Read the model definition and answer for the solid it produces. Units are mm, in the model's axes. A direction names the side the tool comes from. Coordinates: 2 decimals unless noted, no trailing zeros. Order: outer loops, then holes, each group sorted by start corner. A loop starts at its lowest first (then second) coordinate and runs counter-clockwise, first axis right, second up. Notation, with made-up numbers: (23, 85) - (50, 85) arc R17 ccw to (50, 108) - close; hole circle Ø1 at (-22.5, 69). An arc over 180 degrees is marked (long way). Write item = value, one per line.
from build123d import *

# Parameters (mm, degrees)
SKETCH1_W           = 25.9
SKETCH1_H           = 30
BOSS_EXTRUDE1_DEPTH = 7
BOSS_EXTRUDE2_DEPTH = 10
CUT_EXTRUDE1_DEPTH  = 10
SKETCH4_W           = 25.9
SKETCH4_H           = 7
BOSS_EXTRUDE3_DEPTH = 12


with BuildPart() as part:
    # Sketch1 → Boss-Extrude1 (new body)
    with BuildSketch(Plane.XY):
        with Locations((-0.908401305, 7.099021207)):
            Rectangle(SKETCH1_W, SKETCH1_H)
    extrude(amount=BOSS_EXTRUDE1_DEPTH)

    # Sketch2 → Boss-Extrude2 (add)
    with BuildSketch(Plane(origin=(0, 22.099021207, 0), x_dir=(1, 0, 0), z_dir=(0, 1, 0))):
        Polygon((-13.858401305, -4.5), (-16.158401305, -5.116283143), (-16.158401305, -1.733716857), (-13.858401305, -2.35), align=None)
        Polygon((12.041598695, -2.35), (14.341598695, -1.733716857), (14.341598695, -5.116283143), (12.041598695, -4.5), align=None)
    extrude(amount=-BOSS_EXTRUDE2_DEPTH)

    # Sketch3 → Cut-Extrude1 (cut)
    with BuildSketch(Plane(origin=(0, 0, 0), x_dir=(-1, 0, 0), z_dir=(0, 0, -1))):
        with BuildLine():
            Line((-3.791598695, 10.666053203), (-3.791598695, 22.099021207))
            Line((-3.791598695, 22.099021207), (5.608401305, 22.099021207))
            Line((5.608401305, 22.099021207), (5.608401305, 10.666053203))
            ThreePointArc((5.608401305, 10.666053203), (0.908401305, 5.966053203), (-3.791598695, 10.666053203))
        make_face()
    extrude(amount=-CUT_EXTRUDE1_DEPTH, mode=Mode.SUBTRACT)

    # Sketch4 → Boss-Extrude3 (add)
    with BuildSketch(Plane.XZ.offset(7.900978793)):
        with Locations((-0.908401305, 3.5)):
            Rectangle(SKETCH4_W, SKETCH4_H)
    extrude(amount=BOSS_EXTRUDE3_DEPTH)


solid = part.part
1) The part is cut by section C-C (z = 0.5). Determine the outline of the cut face in (x, y), and give its area (3 significant figures).
Returned:
outline = (-13.86, -19.9) - (12.04, -19.9) - (12.04, 22.1) - (3.79, 22.1) - (3.79, 10.67) arc R4.7 cw to (-5.61, 10.67) - (-5.61, 22.1) - (-13.86, 22.1) - close
area = 946 mm^2
2) For faces 5 (the face through (-5.608, 16, 3)), 6 (the face through (-15, 12.099, 3)), 7 (the face through (13.175, 17.169, 2.046)), 8 (the face through (-1, 1, 0)), 9 (the face through (13.208, 17.169, 4.812)), determine the directions among +Z, -Z, +X, -X, +Y, -Y from which every point of the face is accessible in a straight line to the end or side of a thin tool.
Returned:
face_5 = +Z, -Z, +Y
face_6 = +Z, -Z, -X, -Y
face_7 = -Z, +Y, -Y
face_8 = -Z, +X, -X, +Y, -Y
face_9 = +Z, +Y, -Y
3) Determine the mould class of faces 1 (the face through (14.342, 17, 3)), 2 (the face through (-16.158, 17, 3)), 3 (the face through (13, 12.099, 3)), 4 (the face through (3.792, 16, 3)) for opening direction X: pulls with the +X half, pulls with the -X half, needs draft (parallel to the pull), parting line crosses it, or undercut.
Returned:
face_1 = pulls with the +X half
face_2 = pulls with the -X half
face_3 = needs draft
face_4 = undercut
4) The part is cut by section B-B (y = -10). Determine the outline of the cut face in (x, z), and give its area (3 significant figures).
Returned:
outline = (-13.86, 0) - (12.04, 0) - (12.04, 7) - (-13.86, 7) - close
area = 181 mm^2
5) Flat-ended cylindrical pins translate along their axes: pin 1 Ø2.5 at (x, z) = (-15, 3.5) entering from -Y; pin 2 Ø2 at (y, z) = (11, 2.5) entering from -X; pin 3 Ø0.7 at (x, z) = (13, 3.5) entering from -Y. Find the tip coordinate at first contact, or state that the pin passes through.
Returned:
pin_1 = -19.9
pin_2 = -13.86
pin_3 = 12.1
6) The part is cut by section D-D (x = 1.5). Determine the outline of the cut face in (y, z).
Returned:
outline = (-19.9, 0) - (6.63, 0) - (6.63, 7) - (-19.9, 7) - close
7) Straight lines are drawn through the part: line 1 along X through (y, z) = (15, 3.75); line 2 along Y through (x, z) = (13.5, 4.5); line 3 along X through (y, z) = (-12, 5.75). For each, find the intervals that lie inside material, in ascending order. Write a range as from..to.
Returned:
line_1 = -16.16..-5.61, 3.79..14.34
line_2 = 12.1..22.1
line_3 = -13.86..12.04
8) The part is cut by section A-A (z = 3). Determine the outline of the cut face in (x, y).
Returned:
outline = (-16.16, 12.1) - (-13.86, 12.1) - (-13.86, -19.9) - (12.04, -19.9) - (12.04, 12.1) - (14.34, 12.1) - (14.34, 22.1) - (3.79, 22.1) - (3.79, 10.67) arc R4.7 cw to (-5.61, 10.67) - (-5.61, 22.1) - (-16.16, 22.1) - close
